Input: dimensioned drawing with shaded views. Units: mm. Origin: part minimum x, y, z. A direction names the side the tool comes from. Give positions to 0.01 mm unless a question says otherwise; leave off trailing zeros. Write each loop counter-clockwise with the first axis right and the second up, starting at its lowest first coordinate (ties: lowest second). Pieces come first, ordered by that corner, then holes. Notation, with made-up numbers: (22, 65.25) -> (78, 65.25) arc R29 ccw to (78, 85.25) -> close; hole circle Ø6 at (65.25, 28). An arc over 180 degrees is marked (long way). Answer as a JSON object with one key per item and string values. Group by question number.
(1) Draft query along Y for the marked faces 1, 2 and 3. Return one class per face: +Y half, -Y half, draft (parallel to the pull), parting line (faces both ways), or undercut.
(2) Set-up query: the marked faces 4, 5, 6, 7 and 8. Return all of +Z, -Z, +X, -X, +Y, -Y with unobstructed straight access to the full face (end or side cutting, diameter ignored); none if empty.
(3) Section query A-A on x = 38.1. Output: boundary loops of the cut face in (y, z) (3 decimals), plus the area to 3 significant figures.
(4) Contact query for flat-ended pins moving along their axis: pin 1 Ø3 at (x, z) = (69, 7.5) entering from -Y (3 decimals); pin 2 Ø4 at (y, z) = (21.5, 6) entering from -X (3 decimals); pin 3 Ø1.5 at (x, y) = (40.5, 38.5) entering from +Z (3 decimals). Output: stop coordinate, or through.
(5) Section query C-C on z = 10. Output: boundary loops of the cut face in (x, y) (3 decimals), plus the area to 3 significant figures.
(6) Material intervals for probe 1 along Y at (x, z) = (38.1, 10.25) (3 decimals); probe 2 along Z at (x, y) = (37, 45.5) (3 decimals); probe 3 along X at (y, z) = (29, 2.5) (3 decimals), sorted ascending.
(7) Section query B-B on y = 18. Output: boundary loops of the cut face in (x, z) (3 decimals).
(8) Section query D-D on x = 71. Output: boundary loops of the cut face in (y, z) (3 decimals), plus the area to 3 significant figures.
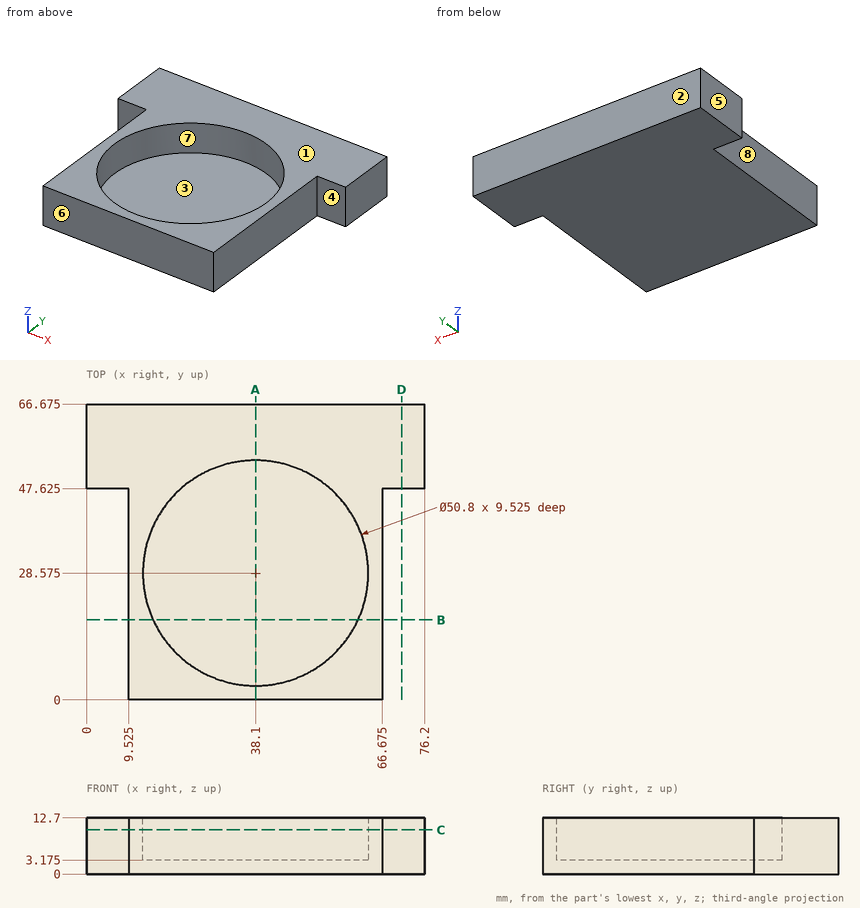
Answer list:
{
 "1": {"face 1": "draft", "face 2": "+Y half", "face 3": "undercut"},
 "2": {"face 4": "+Z, -Z, +X, -Y", "face 5": "+Z, -Z, -X, +Y, -Y", "face 6": "+Z, -Z, +X, -X, -Y", "face 7": "+Z", "face 8": "+Z, -Z, -X, -Y"},
 "3": {"outline": "(0, 0) -> (66.675, 0) -> (66.675, 12.7) -> (53.975, 12.7) -> (53.975, 3.175) -> (3.175, 3.175) -> (3.175, 12.7) -> (0, 12.7) -> close", "area": "363 mm2"},
 "4": {"pin 1": "y = 47.625", "pin 2": "x = 9.525", "pin 3": "z = 3.175"},
 "5": {"outline": "(0, 47.625) -> (9.525, 47.625) -> (9.525, 0) -> (66.675, 0) -> (66.675, 47.625) -> (76.2, 47.625) -> (76.2, 66.675) -> (0, 66.675) -> close; hole circle Ø50.8 at (38.1, 28.575)", "area": "2,150 mm2"},
 "6": {"probe 1": "0 to 3.175, 53.975 to 66.675", "probe 2": "0 to 3.175", "probe 3": "9.525 to 66.675"},
 "7": {"outline": "(9.525, 0) -> (66.675, 0) -> (66.675, 12.7) -> (61.194, 12.7) -> (61.194, 3.175) -> (15.006, 3.175) -> (15.006, 12.7) -> (9.525, 12.7) -> close"},
 "8": {"outline": "(47.625, 0) -> (66.675, 0) -> (66.675, 12.7) -> (47.625, 12.7) -> close", "area": "242 mm2"}
}
